Autodesk Inventor part; units mm, degrees
ref_plane "YZ Plane" through (0, 0, 0) normal (1, 0, 0) x (0, 1, 0)
ref_plane "XZ Plane" through (0, 0, 0) normal (0, 1, 0) x (-1, 0, 0)
ref_plane "XY Plane" through (0, 0, 0) normal (0, 0, 1) x (1, 0, 0)
sketch "Sketch1" plane through (0, 0, 0) normal (0, 0, 1) x (1, 0, 0)
  line L0 (440.770723, -684.385341) -> (440.770723, -734.385341) construction
  line L1 (0, 47) -> (0, 0) construction
  arc A0 (0.159434, 1.869277) -> (0, 1880) centre (-11009.945504, 940) ccw
  arc A1 (0, 0) -> (0.159434, 1.869277) centre (-11009.945504, 940) ccw construction
  arc A2 (-1.349222, -1.302929) -> (0.159434, 1.869277) centre (-4.822514, 2.29377) ccw
  line L2 (-1.349222, -1.302929) -> (0, 0) construction
  line L3 (-46.757087, -45.152794) -> (-1.349222, -1.302929)
  line L4 (-41.190716, -50.91694) -> (-46.757087, -45.152794) construction
  line L5 (0, 0) -> (0, 1880) construction
  line L6 (0, 0) -> (1.875639, 0) construction
  dimension "d154" = 5
  dimension "d155" = 65
  dimension "d156" = 11050
  dimension "d157" = 136
  dimension "d158" = 1880
contour flange "Contour Flange2" sketch "Sketch1" thickness 3 bend radius 3 width 980 along (0, 0, 1) mid plane no both sides no wall seen from (-24.053155, -23.227861, 0) lies toward (0.6946584, -0.7193398, 0) curves L3 A2 A0
bend "Bend2"
corner "Corner2"
sketch "Sketch6" plane through (0, 0, 0) normal (1, 0, 0) x (0, 1, 0)
  line L0 (1.869277, 0) -> (1.869277, 980)
  line L1 (1880, 980) -> (1.869277, 980)
  line L2 (1.869277, 0) -> (1880, 0)
  line L3 (1880.255204, 980) -> (1880, 980)
  line L4 (1880.255204, 0) -> (1880.255204, 980)
  line L5 (1880.255204, 0) -> (1880, 0)
  line L6 (1238.553761, 0) -> (1880.255204, 764.75)
  line L7 (1880.255204, 215.25) -> (1238.553761, 980)
  point P0 (0, 0)
  dimension "d160" = 40
  dimension "d161" = 215.25
extrude "Extrusion3" cut sketch "Sketch6" along normal through all both and the other way through all contours L1 L3 L4 L6 L7 | L6 L4 L7
sketch "Sketch7" plane through (-1.349222, -1.302929, 980) normal (-0.6946584, 0.7193398, 0) x (0.7193398, 0.6946584, 0)
  line L0 (-83.025107, 17.798613) -> (-83.025107, 187.19296) construction
  line L1 (-83.025107, 187.19296) -> (-68.508178, 187.19296) construction
  line L2 (-68.508178, 187.19296) -> (-68.508178, 17.798613) construction
  line L3 (-68.508178, 17.798613) -> (-83.025107, 17.798613) construction
  point P0 (1.875639, 980)
feature "Mark5" [suppressed]
equation "\"d36\" = Thickness"
equation "\"d37\" = BendReliefWidth"
equation "\"d38\" = BendReliefDepth"
equation "\"d39\" = MinimumRemnant"
equation "\"d40\" = TransitionRadius"
equation "\"d42\" = BendRadius"
equation "\"d44\" = CornerReliefSize"
equation "\"d45\" = GapSize"
equation "\"d46\" = JacobiRadiusSize"
equation "\"BendRadius\" = Thickness"
equation "\"BendReliefWidth\" = Thickness"
equation "\"BendReliefDepth\" = 0.5 * Thickness"
equation "\"CornerReliefSize\" = 4 * Thickness"
equation "\"MinimumRemnant\" = 2 * Thickness"
equation "\"TransitionRadius\" = BendRadius"
equation "\"JacobiRadiusSize\" = BendRadius"
equation "\"GapSize\" = Thickness"
properties part number "MSC 310 sheet left board withers" material "AISI304"
Geometry: final body of the model. Coordinates: model frame, mm. Give positions to 0.01 mm unless a question says otherwise; leave off trailing zeros. Order: outer loops, then holes, each group sorted by start corner. A loop starts at its lowest first (then second) coordinate and runs counter-clockwise, first axis right, second up. Notation, with made-up numbers: (-17, 22.5) -> (2, 22.5) arc R15 ccw to (2, 34.5) -> close; hole circle Ø1 at (31.25, 85). An arc over 180 degrees is marked (long way). Answer as a JSON object with one key per item and string values.
Q1. Draft query along Y for faces 1 (the cylindrical face through (41.336, 745.125, 483.14)), 2 (the cylindrical face through (38.337, 745.178, 483.14)), 3 (the flat face through (-22.287, -25.693, 483.14)), 4 (the flat face through (-24.371, -23.535, 483.14)). Return one class per face: released by +Y, released by -Y, zero draft, split by the parting line, or undercut.
Entries:
{"face 1": "split by the parting line", "face 2": "undercut", "face 3": "released by -Y", "face 4": "released by +Y"}
Q2. First-contact query: pin 1 (10 mm diameter, centred on y = 337.5, z = 800, fed in from +X). Flat tip, straight axial feed; report the tip coordinate or a pass-through.
Entries:
{"pin 1": "stops at x = 26.89"}
Q3. Section B-B (z = 867). Output: boundary loops of the cut face in (x, y).
Entries:
{"outline": "(-46.76, -45.15) -> (-44.67, -47.31) -> (0.73, -3.46) arc R8 ccw to (3.15, 1.61) arc R11053 ccw to (36.05, 1333.37) -> (33.05, 1333.37) arc R11050 cw to (0.16, 1.87) arc R5 cw to (-1.35, -1.3) -> close"}
Q4. Section C-C (y = 231.5). Output: boundary loops of the cut face in (x, z), plus the area to 3 significant figures.
Entries:
{"outline": "(17.32, 0) -> (20.32, 0) -> (20.32, 980) -> (17.32, 980) -> close", "area": "2,950 mm^2"}
Q5. Material intervals for probe 1 along X at (y, z) = (879, 204.5); probe 2 along Z at (x, y) = (11, 1776); probe 3 along Y at (x, z) = (-41.5, 256.5), sorted ascending.
Entries:
{"probe 1": "x = 39.89 to 42.89", "probe 2": "z = 0 to 339.5", "probe 3": "y = -44.25 to -40.08"}
Q6. Section D-D (z = 633). Output: boundary loops of the cut face in (x, y).
Entries:
{"outline": "(-46.76, -45.15) -> (-44.67, -47.31) -> (0.73, -3.46) arc R8 ccw to (3.15, 1.61) arc R11053 ccw to (27.31, 1529.72) -> (24.31, 1529.72) arc R11050 cw to (0.16, 1.87) arc R5 cw to (-1.35, -1.3) -> close"}
